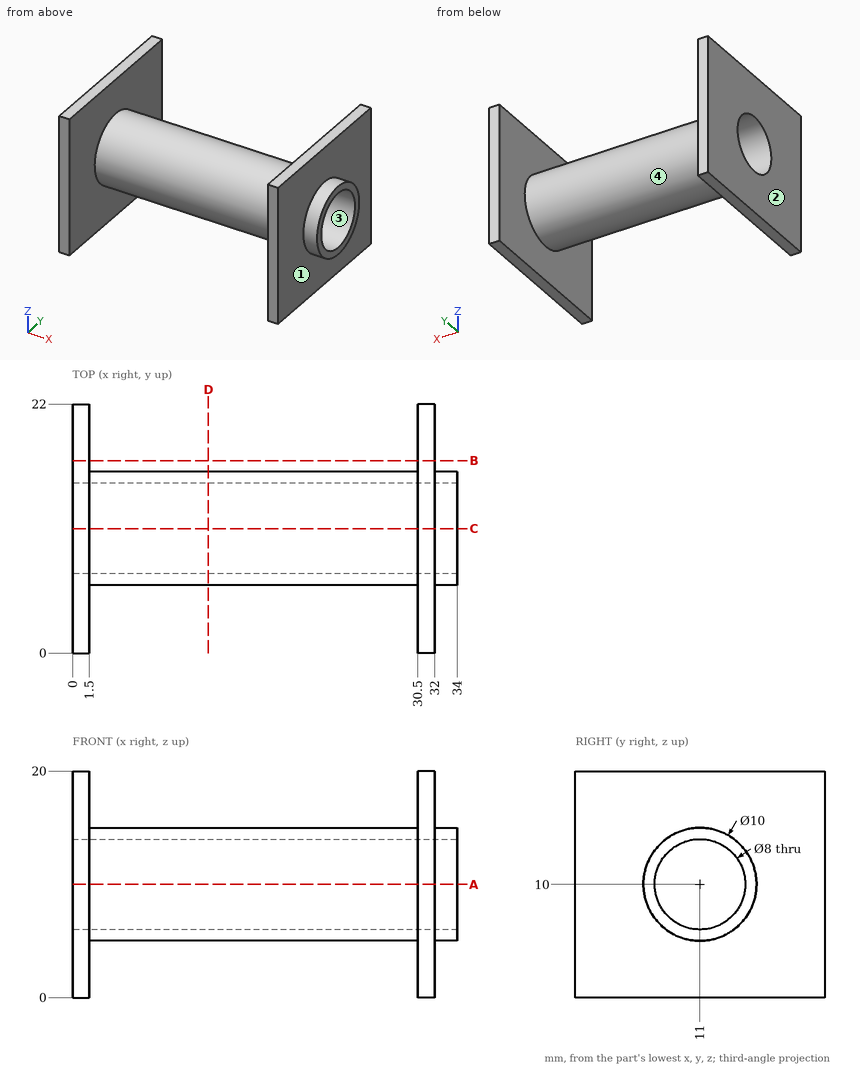
Geometry check sheet. Reference: drawing and pictorial views, mm from the part's lowest x, y, z. Round coordinates to 2 decimals unless told otherwise and drop trailing zeros. Write each loop counter-clockwise with the first axis right and the second up, starting at its lowest first coordinate (ties: lowest second). Pieces come first, ordered by that corner, then holes. Notation, with made-up numbers: (59.5, 46) -> (110.5, 46) arc R10 cw to (110.5, 52) -> close; hole circle Ø11 at (22, 42.25). An arc over 180 degrees is marked (long way). Put each result on its own line as item: value.
1) Cross-section at B-B, the plane y = 17. Enter the section's corners in (x, z), plus the area to 3 significant figures.
Recorded:
outline: (0, 0) -> (1.5, 0) -> (1.5, 20) -> (0, 20) -> close; (30.5, 0) -> (32, 0) -> (32, 20) -> (30.5, 20) -> close
area: 60.0 mm2
2) Cross-section at C-C, the plane y = 11. Enter the section's corners in (x, z), plus the area to 3 significant figures.
Recorded:
outline: (0, 0) -> (1.5, 0) -> (1.5, 5) -> (30.5, 5) -> (30.5, 0) -> (32, 0) -> (32, 5) -> (34, 5) -> (34, 6) -> (0, 6) -> close; (0, 14) -> (34, 14) -> (34, 15) -> (32, 15) -> (32, 20) -> (30.5, 20) -> (30.5, 15) -> (1.5, 15) -> (1.5, 20) -> (0, 20) -> close
area: 98.0 mm2
3) Thickness scan on probe 1 along X at (y, z) = (21.25, 4); probe 2 along Y at (x, z) = (16, 10); probe 3 along Z at (x, y) = (14, 9). Record the ranges inside material, lowest first. Write a range as from..to.
Recorded:
probe 1: x = 0..1.5, 30.5..32
probe 2: y = 6..7, 15..16
probe 3: z = 5.42..6.54, 13.46..14.58
4) Depth check by flat-ended pin: P1, Ø5, axis at x = 19.5, y = 6, coming from the -Z side; P2, Ø8, axis at x = 13.5, y = 18, coming from the +Z side; P3, Ø8, axis at x = 26, z = 9.5, coming from the -Y side. Enter the tip coordinate at first touch or a pass-through.
Recorded:
P1: stops at z = 5.67
P2: stops at z = 14
P3: stops at y = 6
5) Cross-section at D-D, the plane x = 12. Enter the section's corners in (y, z).
Recorded:
outline: circle Ø10 at (11, 10); hole circle Ø8 at (11, 10)
6) Release check for a two-part mould opening along X. For the marked faces 1, 2, 3 and 4 record: pulls with the +X half, pulls with the -X half, needs draft (parallel to the pull), parting line crosses it, or undercut.
Recorded:
face 1: pulls with the +X half
face 2: pulls with the -X half
face 3: needs draft
face 4: undercut
7) Cross-section at A-A, the plane z = 10. Enter the section's corners in (x, y).
Recorded:
outline: (0, 0) -> (1.5, 0) -> (1.5, 6) -> (30.5, 6) -> (30.5, 0) -> (32, 0) -> (32, 6) -> (34, 6) -> (34, 7) -> (0, 7) -> close; (0, 15) -> (34, 15) -> (34, 16) -> (32, 16) -> (32, 22) -> (30.5, 22) -> (30.5, 16) -> (1.5, 16) -> (1.5, 22) -> (0, 22) -> close
